Input: part model. Units: mm. Frame: model coordinates. A direction names the side the tool comes from. Round coordinates to 2 decimals unless told otherwise and drop trailing zeros. Order: outer loops, then holes, each group sorted by start corner. A loop starts at its lowest first (then second) coordinate and runs counter-clockwise, first axis right, second up. Notation, with made-up numbers: (39.25, -16.5) -> (74.25, -16.5) arc R23 ccw to (74.25, 6.5) -> close; hole circle Ø8 at (-2, 88). An arc over 180 degrees is marked (long way). Use a Markdown table: item, result.
Autodesk Inventor part; units mm, degrees
ref_plane "YZ Plane" through (0, 0, 0) normal (1, 0, 0) x (0, 1, 0)
ref_plane "XZ Plane" through (0, 0, 0) normal (0, 1, 0) x (-1, 0, 0)
ref_plane "XY Plane" through (0, 0, 0) normal (0, 0, 1) x (1, 0, 0)
sketch "スケッチ1" plane through (0, 0, 0) normal (0, 1, 0) x (-1, 0, 0)
  line L0 (180, 60) -> (-180, 60)
  line L1 (-180, 60) -> (-180, -60)
  line L2 (-180, -60) -> (180, -60)
  line L3 (180, -60) -> (180, 60)
  line L4 (180, 60) -> (-180, -60) construction
  line L5 (-180, 60) -> (180, -60) construction
  line L6 (180, 57) -> (-180, 57)
  line L7 (-60, 60) -> (-60, -60)
  line L8 (-60, 40) -> (-80, 40)
  line L9 (-80, 40) -> (-80, 20)
  line L10 (-80, 20) -> (-60, 20)
  line L11 (252, 0) -> (-252, 0) construction
  line L12 (-60, -40) -> (-80, -40)
  line L13 (-80, -40) -> (-80, -20)
  line L14 (-80, -20) -> (-60, -20)
  line L15 (0, -84) -> (0, 84) construction
  line L16 (60, 60) -> (60, -60)
  line L17 (60, 40) -> (80, 40)
  line L18 (80, 40) -> (80, 20)
  line L19 (80, 20) -> (60, 20)
  line L20 (60, -40) -> (80, -40)
  line L21 (80, -20) -> (60, -20)
  line L22 (80, -40) -> (80, -20)
  line L23 (-60, 19.7) -> (-80.3, 19.7)
  line L24 (-80.3, 19.7) -> (-80.3, 40.3)
  line L25 (-80.3, 40.3) -> (-60, 40.3)
  line L26 (-60, -19.7) -> (-80.3, -19.7)
  line L27 (-80.3, -19.7) -> (-80.3, -40.3)
  line L28 (-80.3, -40.3) -> (-60, -40.3)
  line L29 (60, 19.7) -> (80.3, 19.7)
  line L30 (80.3, 19.7) -> (80.3, 40.3)
  line L31 (80.3, 40.3) -> (60, 40.3)
  line L32 (60, -19.7) -> (80.3, -19.7)
  line L33 (80.3, -19.7) -> (80.3, -40.3)
  line L34 (80.3, -40.3) -> (60, -40.3)
  point P0 (0, 0)
  point P1 (60, 57)
  point P2 (-60, 57)
  dimension "d0" = 120
  dimension "d1" = 360
  dimension "d4" = 3
  dimension "d5" = 120
  dimension "d7" = 20
  dimension "d8" = 20
  dimension "d9" = 20
  dimension "d10" = 0.3
  dimension "d11" = 0.3
extrude "押し出し3" add sketch "スケッチ1" along normal blind 25 contours L3 L6 L16 L0 | L16 L6 L7 L0 | L7 L6 L1 L0
sketch "スケッチ2" plane through (-180, 0, 60) normal (0, 0, 1) x (1, 0, 0)
  line L0 (0, 0) -> (360, 0)
  line L1 (360, 0) -> (360, 25)
  line L2 (0, 25) -> (360, 25)
  line L3 (0, 0) -> (0, 25)
  line L4 (240, 0) -> (240, 25)
  line L5 (240, 7.5) -> (255, 7.5)
  line L6 (255, 7.5) -> (255, 17.5)
  line L7 (255, 17.5) -> (240, 17.5)
  line L8 (180, -5) -> (180, 30) construction
  line L9 (120, 0) -> (120, 25)
  line L10 (120, 7.5) -> (105, 7.5)
  line L11 (105, 7.5) -> (105, 17.5)
  line L12 (105, 17.5) -> (120, 17.5)
  line L13 (240, 17.9) -> (255.4, 17.9)
  line L14 (255.4, 17.9) -> (255.4, 7.1)
  line L15 (255.4, 7.1) -> (240, 7.1)
  line L16 (120, 17.9) -> (104.6, 17.9)
  line L17 (104.6, 17.9) -> (104.6, 7.1)
  line L18 (104.6, 7.1) -> (120, 7.1)
  point P0 (180, 0)
  point P1 (360, 12.5)
  dimension "d16" = 120
  dimension "d17" = 10
  dimension "d18" = 15
  dimension "d19" = 7.5
  dimension "d24" = 0.4
extrude "押し出し6" add sketch "スケッチ1" along normal blind 2 contours L16 L2 L7 L6
extrude "押し出し7" add sketch "スケッチ1" against normal blind 1 from surface at 2 contours L17 L18 L19 L16 | L7 L10 L9 L8 | L16 L21 L22 L20 | L12 L13 L14 L7
extrude "押し出し8" cut sketch "スケッチ2" against normal up to surface (3 mm away) contours L3 L2 L9 L16 L17 L18 L0 | L4 L15 L14 L13 L2 L1 L0 | L18 L17 L16 L9 L12 L11 L10 | L4 L5 L6 L7 L13 L14 L15 | L10 L11 L12 L9 | L4 L7 L6 L5
fillet "フィレット2" radius 1 1 edges at (0, 2, -60)
extrude "押し出し9" add sketch "スケッチ2" against normal blind 1 contours L10 L11 L12 L9 | L4 L7 L6 L5
fillet "フィレット3" radius 4 1 edges at (0, 2, 57)
properties part number "protectar1"
1) Cut plane A-A on x = -67. Return loops of the section in (y, z).
Results found:
| item | result |
|---|---|
| outline | (1, -40) -> (2, -40) -> (2, -20) -> (1, -20) -> close; (1, 20) -> (2, 20) -> (2, 40) -> (1, 40) -> close; (7.5, 59) -> (17.5, 59) -> (17.5, 60) -> (7.5, 60) -> close |
2) Pull-direction query (Z, two-part tool) for faces 1 (the flat face through (-68, 13, 59)), 2 (the flat face through (-70, 1, 30)), 3 (the flat face through (-60, 0.4, 22.5)); classes: +Z half, -Z half, draft (parallel to the pull), parting line (faces both ways), or undercut.
Results found:
| item | result |
|---|---|
| face 1 | -Z half |
| face 2 | draft |
| face 3 | undercut |
3) Cut plane B-B on x = -21. Return loops of the section in (y, z), and give its area (3 significant figures).
Results found:
| item | result |
|---|---|
| outline | (0, -60) -> (1, -60) arc R1 ccw to (2, -59) -> (2, 53) arc R4 cw to (6, 57) -> (25, 57) -> (25, 60) -> (0, 60) -> close |
| area | 312 mm² |
4) Pin query (flat end, axial travel): pin 1 Ø16 at (x, z) = (-69, 29) entering from -Y; pin 2 Ø2 at (x, z) = (-56.5, -0.5) entering from +Y; pin 3 Ø1.1 at (y, z) = (13.5, 59.5) entering from -X. Return the tip coordinate at first contact, or that it passes through.
Results found:
| item | result |
|---|---|
| pin 1 | stops at y = 1 |
| pin 2 | stops at y = 2 |
| pin 3 | stops at x = -75 |
5) Set-up query: faces 4 (the flat face through (67, 13, 59)), 5 (the flat face through (70, 1, 30)), 6 (the flat face through (-1, 15, 57)). Return all of +Z, -Z, +X, -X, +Y, -Y with unobstructed straight access to the full face (end or side cutting, diameter ignored); none if empty.
Results found:
| item | result |
|---|---|
| face 4 | -Z, +X, +Y, -Y |
| face 5 | +Z, -Z, +X, -Y |
| face 6 | -Z, +X, -X, +Y |
6) Cut plane C-C on y = 13. Return loops of the section in (x, z).
Results found:
| item | result |
|---|---|
| outline | (-75, 59) -> (-60, 59) -> (-60, 57) -> (60, 57) -> (60, 59) -> (75, 59) -> (75, 60) -> (-75, 60) -> close |
7) Cut plane D-D on z = 43. Return loops of the section in (x, y).
Results found:
| item | result |
|---|---|
| outline | (-60, 0) -> (60, 0) -> (60, 2) -> (-60, 2) -> close |
8) Line query: L1, parallel to Z at x = 62, y = 1.5; L2, parallel to Y at x = -65, z = -21; L3, parallel to Y at x = -0.5, z = -36. Output: solid intervals per line, ascending. Write a range as [from, to].
Results found:
| item | result |
|---|---|
| L1 | z = [-40, -20], [20, 40] |
| L2 | y = [1, 2] |
| L3 | y = [0, 2] |
